Model file for the job. Use its own axes, mm. A direction names the side the tool comes from. Give positions to 0.01 mm unless a question says otherwise; leave off trailing zeros. Loops run counter-clockwise (first coordinate to the right, second up) from the corner with the lowest first, then second, coordinate; pieces in that order, holes last. Notation, with made-up numbers: M 18.5,-40 L 69.5,-40 A14 cw 69.5,-24 Z; hole C 37.25,-4 d2. An arc over 180 degrees is marked long. Answer in a Markdown table with one row per item.
```python
from build123d import *

# Parameters (mm, degrees)
F0_W           = 127
F0_H           = 101.6
F1_DEPTH       = 76.2
F3_D           = 11
F3_CBORE_D     = 17.25
F3_CBORE_DEPTH = 10
F4_SIZE        = 5.08
F5_R           = 12.7
F6_T           = -5.08


with BuildPart() as f1:
    # F0 (on Front) → F1 (new body)
    with BuildSketch(Plane.XZ):
        with Locations((38.1, -25.4)):
            Rectangle(F0_W, F0_H)
    extrude(amount=F1_DEPTH)

    # F3 (through all)
    with Locations(Plane.XZ.offset(76.2)):
        with Locations((38.1, -25.4)):
            CounterBoreHole(F3_D / 2, F3_CBORE_D / 2, F3_CBORE_DEPTH)

    # F4
    f4_edges = [f1.edges().sort_by_distance(p)[0] for p in [
        (38.1, -76.2, -76.2),
        (101.6, -76.2, -25.4),
    ]]
    chamfer(f4_edges, length=F4_SIZE)

    # F5
    f5_edges = [f1.edges().sort_by_distance(p)[0] for p in [
        (101.6, -35.56, -76.2),
    ]]
    fillet(f5_edges, radius=F5_R)

    # F6
    f6_openings = [f1.faces().sort_by_distance(p)[0] for p in [
        (35.56, -76.2, 23.844989),
    ]]
    offset(amount=F6_T, openings=f6_openings, kind=Kind.INTERSECTION)


solid = f1.part
```
Q1. Saw through at D-D (x = 21). Give the cut face in (y, z), and give its area (3 significant figures).
Reported:
| item | result |
|---|---|
| outline | M -76.2,-71.12 L -71.12,-76.2 L 0,-76.2 L 0,25.4 L -76.2,25.4 L -76.2,20.32 L -5.08,20.32 L -5.08,-71.12 L -69.02,-71.12 L -76.2,-63.94 Z |
| area | 1,250 mm² |
Q2. 3-axis set-ups, long thin cutter, end or side, ignore diameter. For faces 4 (the face through (31.743, -71.27, -19.571)), 5 (the face through (99.1, -73.62, -24.23)), 6 (the face through (42.1, -61.12, -35.5)): which of +Z, -Z, +X, -X, +Y, -Y reach the whole face in a straight line?
Reported:
| item | result |
|---|---|
| face 4 | -Y |
| face 5 | +Z, -Z, +X, -Y |
| face 6 | none |
Q3. Drop flat-ended pins along their axis: pin 1 (2 mm diameter, centred on x = 52.5, z = -56.5, fed in from -Y); pin 2 (10 mm diameter, centred on x = 44, z = -46, fed in from +Y); pin 3 (5 mm diameter, centred on x = 42, z = -22.5, fed in from -Y). Give the stop position or say it passes through.
Reported:
| item | result |
|---|---|
| pin 1 | y = -5.08 |
| pin 2 | y = 0 |
| pin 3 | y = -66.2 |
Q4. Probe probe 1 along X at (y, z) = (-18, -25); probe 2 along Z at (x, y) = (38, -22); probe 3 along Z at (x, y) = (68.5, -19.5). List the from-to ranges inside material, lowest first.
Reported:
| item | result |
|---|---|
| probe 1 | -25.4 to -20.32, 27.53 to 32.61, 43.59 to 48.67, 96.52 to 101.6 |
| probe 2 | -76.2 to -71.12, -35.98 to -30.9, -19.9 to -14.82, 20.32 to 25.4 |
| probe 3 | -76.2 to -71.12, 20.32 to 25.4 |
Q5. Saw through at B-B (x = 38.1). Give the cut face in (y, z) (3 decimals).
Reported:
| item | result |
|---|---|
| outline | M -76.2,-71.12 L -71.12,-76.2 L 0,-76.2 L 0,-30.9 L -66.2,-30.9 L -66.2,-34.025 L -76.2,-34.025 L -76.2,-39.105 L -61.12,-39.105 L -61.12,-35.98 L -5.08,-35.98 L -5.08,-71.12 L -69.016,-71.12 L -76.2,-63.936 Z; M -76.2,-16.775 L -66.2,-16.775 L -66.2,-19.9 L 0,-19.9 L 0,25.4 L -76.2,25.4 L -76.2,20.32 L -5.08,20.32 L -5.08,-14.82 L -61.12,-14.82 L -61.12,-11.695 L -76.2,-11.695 Z |
Q6. Saw through at C-C (z = -25.4). Give the cut face in (x, y) (3 decimals), and give its area (3 significant figures).
Reported:
| item | result |
|---|---|
| outline | M -25.4,-76.2 L -20.32,-76.2 L -20.32,-5.08 L 27.52,-5.08 L 27.52,-61.12 L 24.395,-61.12 L 24.395,-76.2 L 29.475,-76.2 L 29.475,-66.2 L 32.6,-66.2 L 32.6,0 L -25.4,0 Z; M 43.6,-66.2 L 46.725,-66.2 L 46.725,-76.2 L 51.805,-76.2 L 51.805,-61.12 L 48.68,-61.12 L 48.68,-5.08 L 96.52,-5.08 L 96.52,-69.016 L 89.336,-76.2 L 96.52,-76.2 L 101.6,-71.12 L 101.6,0 L 43.6,0 Z |
| area | 2,080 mm² |
Q7. Saw through at A-A (y = -53). Give the cut face in (x, z), and give its area (3 significant figures).
Reported:
| item | result |
|---|---|
| outline | M -25.4,-76.2 L 88.9,-76.2 A12.7 ccw 101.6,-63.5 L 101.6,25.4 L -25.4,25.4 Z; C 38.1,-25.4 d21.16; hole M -20.32,-71.12 L 88.9,-71.12 A7.62 ccw 96.52,-63.5 L 96.52,20.32 L -20.32,20.32 Z; hole C 38.1,-25.4 d11 |
| area | 2,450 mm² |
Q8. Mould opens along Y. For faces 1 (the face through (36.182, -72.658, -67.478)), 2 (the face through (101.6, -35, -20)), 3 (the face through (37, 0, -13)) say: released by +Y, released by -Y, zero draft, split by the parting line, or undercut.
Reported:
| item | result |
|---|---|
| face 1 | undercut |
| face 2 | zero draft |
| face 3 | released by +Y |
